Geometry check sheet. Reference: the model listing, model coordinates, mm. Coordinates: 2 decimals unless noted, no trailing zeros. Write each loop counter-clockwise with the first axis right and the second up, starting at its lowest first coordinate (ties: lowest second). Pieces come first, ordered by that corner, then holes. Notation, with made-up numbers: (18.25, 27) -> (72.25, 27) arc R31 cw to (72.25, 58) -> close; hole circle Ø5 at (-8, -16.5). An arc over 180 degrees is marked (long way). Use a Markdown table: item, result.
Autodesk Inventor part; units mm, degrees
ref_plane "YZ Plane" through (0, 0, 0) normal (1, 0, 0) x (0, 1, 0)
ref_plane "XZ Plane" through (0, 0, 0) normal (0, 1, 0) x (-1, 0, 0)
ref_plane "XY Plane" through (0, 0, 0) normal (0, 0, 1) x (1, 0, 0)
sketch "Skizze1" plane through (0, 0, 0) normal (0, 1, 0) x (-1, 0, 0)
  circle A0 centre (0, 0) radius 200
  dimension "d0" = 400
extrude "Extrusion1" add sketch "Skizze1" along normal blind 10
sketch "Skizze2" plane through (0, 10, 0) normal (0, 1, 0) x (1, 0, 0)
  circle A0 centre (0, 0) radius 200
  line L0 (0, 0) -> (200, 0) construction
  line L1 (0, 0) -> (61.8034, 190.2113)
  line L2 (0, 0) -> (200, 0) construction
  line L3 (0, 0) -> (-161.8034, 117.5571)
  line L4 (0, 0) -> (200, 0) construction
  line L5 (0, 0) -> (61.8034, -190.2113)
  line L6 (0, 0) -> (-161.8034, -117.5571)
  line L7 (0, 0) -> (200, 0)
  line L8 (200, 0) -> (100, 0)
  line L9 (0, 0) -> (30.9017, -95.1057)
  line L10 (200, 0) -> (135, 0)
  circle A1 centre (135, 0) radius 50
  line L11 (61.8034, -190.2113) -> (41.7173, -128.3926)
  circle A2 centre (41.7173, -128.3926) radius 50
  line L12 (-161.8034, -117.5571) -> (-109.2173, -79.351)
  circle A3 centre (-109.2173, -79.351) radius 50
  line L13 (-161.8034, 117.5571) -> (-109.2173, 79.351)
  circle A4 centre (-109.2173, 79.351) radius 50
  line L14 (61.8034, 190.2113) -> (41.7173, 128.3926)
  circle A5 centre (41.7173, 128.3926) radius 50
  dimension "d4" = 72
  dimension "d5" = 144
  dimension "d9" = 65
  dimension "d10" = 100
  dimension "d11" = 65
  dimension "d12" = 100
  dimension "d13" = 65
  dimension "d14" = 100
  dimension "d15" = 65
  dimension "d16" = 100
  dimension "d17" = 65
  dimension "d18" = 100
extrude "Extrusion4" cut sketch "Skizze2" against normal blind 10 contours A1 L7 | L7 A1 | A5 L1 | L1 A5 | A2 L5 | L5 A2 | A4 L3 | L3 A4 | A3 L6 | L6 A3
sketch "Skizze5" plane through (0, 0, 0) normal (0, -1, 0) x (1, 0, 0)
  circle A0 centre (0, 0) radius 7.5
  dimension "d27" = 15
extrude "Extrusion5" cut sketch "Skizze5" against normal blind 10
sketch "Skizze6" plane through (0, 0, 0) normal (0, -1, 0) x (1, 0, 0)
  line L0 (0, 0) -> (0, 16.25)
  line L1 (0, 0) -> (15.4547, 5.0215)
  line L2 (0, 0) -> (16.25, 0) construction
  line L3 (0, 0) -> (16.25, 0) construction
  line L4 (0, 0) -> (9.5515, -13.1465)
  line L5 (0, 0) -> (16.25, 0) construction
  line L6 (0, 0) -> (-9.5515, -13.1465)
  line L7 (0, 0) -> (16.25, 0) construction
  line L8 (0, 0) -> (-15.4547, 5.0215)
  dimension "d30" = 16.25
  dimension "d31" = 16.25
  dimension "d32" = 18
  dimension "d35" = 16.25
  dimension "d36" = 54
  dimension "d37" = 16.25
  dimension "d40" = 16.25
hole "Bohrung1" at (0, 0, 16.25) at (-15.4547, 0, 5.0215) at (-9.5515, 0, -13.1465) at (15.4547, 0, 5.0215) at (9.5515, 0, -13.1465) direction (0, 1, 0) diameter 9 depth 10 tip angle 118
properties part number "Drehplatte_Rahmenvorrrichtung" material "Holz (Birke)"
Item 1: Section check B-B on x = 115. Record the boundary of the cut face in (y, z).
Answer block:
| item | result |
|---|---|
| outline | (0, -163.63) -> (10, -163.63) -> (10, -45.83) -> (0, -45.83) -> close; (0, 45.83) -> (10, 45.83) -> (10, 163.63) -> (0, 163.63) -> close |
Item 2: Section check A-A on z = 155.5. Record the boundary of the cut face in (x, y), then the cut area to 3 significant figures.
Answer block:
| item | result |
|---|---|
| outline | (-125.78, 0) -> (-0.3, 0) -> (-0.3, 10) -> (-125.78, 10) -> close; (83.73, 0) -> (125.78, 0) -> (125.78, 10) -> (83.73, 10) -> close |
| area | 1,680 mm^2 |
Item 3: Mould release check, pull along Z, two halves, no side actions. Record for faces 1 (the flat face through (-42, 0, 3)), 2 (the cylindrical face through (-190.764, 4.93, -60.075)), 3 (the cylindrical face through (12.29, 5.07, -9.575)): +Z half, -Z half, draft (parallel to the pull), parting line (faces both ways), or undercut.
Answer block:
| item | result |
|---|---|
| face 1 | draft |
| face 2 | parting line |
| face 3 | undercut |
Item 4: Section check C-C on y = 7. Count the separate pieces of the cut face and the enclosed holes in it, then the cut area to 3 significant figures.
Answer block:
| item | result |
|---|---|
| separate pieces | 1 |
| enclosed holes | 11 |
| area | 85,900 mm^2 |
Item 5: Thickness scan on L1, parallel to X at y = 1, z = -5.5; L2, parallel to X at y = 5.75, z = 16.25; L3, parallel to Z at x = -115, y = 4. Record the ranges inside material, lowest first. Write a range as [from, to].
Answer block:
| item | result |
|---|---|
| L1 | x = [-199.92, -5.1], [5.1, 85.3], [184.7, 199.92] |
| L2 | x = [-199.34, -4.5], [4.5, 87.71], [182.29, 199.34] |
| L3 | z = [-163.63, -129.02], [-29.69, 29.69], [129.02, 163.63] |
Item 6: Depth check by flat-ended pin: P1, Ø1, axis at y = 7, z = -118.5, coming from the -X side; P2, Ø4, axis at y = 1.5, z = -62.5, coming from the +X side; P3, Ø4, axis at x = 121.5, y = 4, coming from the +Z side. Enter the tip coordinate at first touch or a pass-through.
Answer block:
| item | result |
|---|---|
| P1 | stops at x = -161.48 |
| P2 | stops at x = 190.63 |
| P3 | stops at z = 160.37 |
